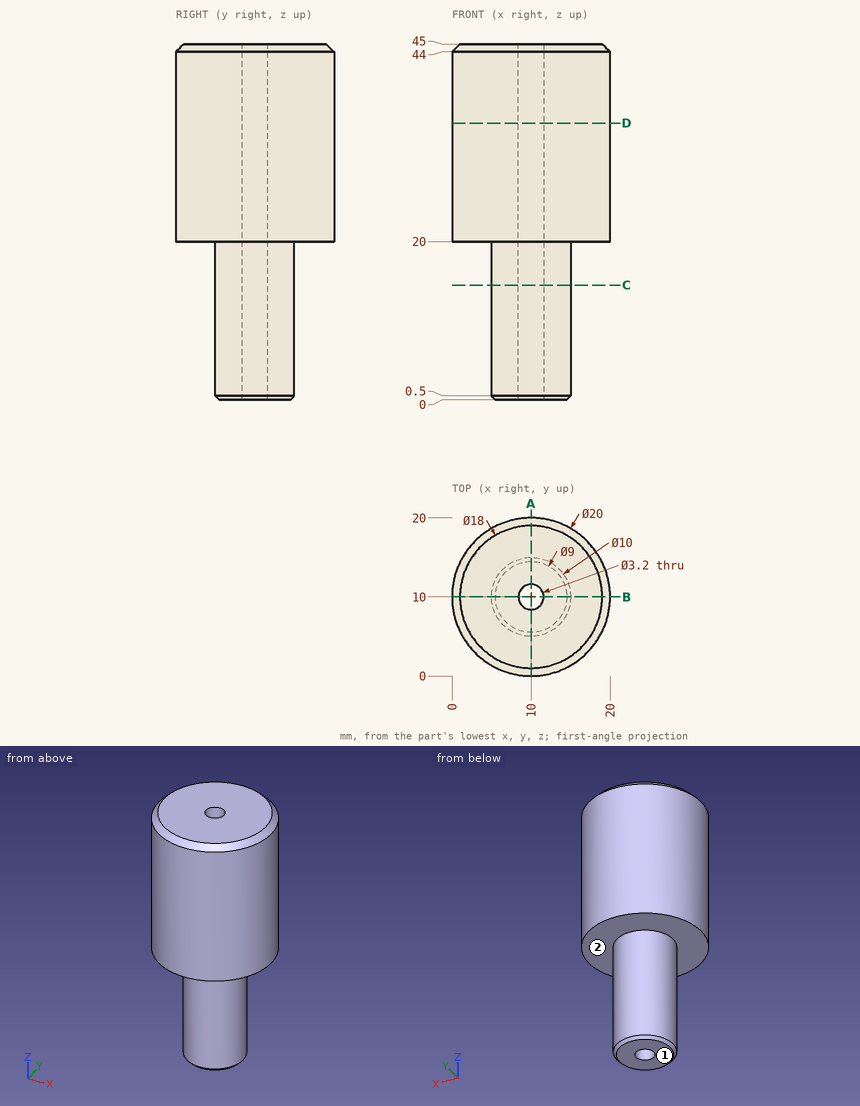
Study the drawing (mm; zero at the part's minimum x, y, z) and answer. A direction names the side the tool comes from. Give positions to 0.01 mm unless a question says otherwise; leave off trailing zeros. Order: outer loops, then holes, each group sorted by start corner. A loop starts at its lowest first (then second) coordinate and runs counter-clockwise, first axis right, second up.
1) For the marked faces 1 and 2, determine the directions among +Z, -Z, +X, -X, +Y, -Y from which every point of the face is accessible in a straight line to the end or side of a thin tool.
Reported:
face 1: -Z, +X, -X, +Y, -Y
face 2: -Z
2) Find section D-D on z = 35. Write down the section's boundary in (x, y), then the cut area to 3 significant figures.
Reported:
outline: circle Ø20 at (10, 10); hole circle Ø3.2 at (10, 10)
area: 306 mm2
3) Find section A-A on x = 10. Write down the section's boundary in (y, z), then the cut area to 3 significant figures.
Reported:
outline: (0, 20) - (5, 20) - (5, 0.5) - (5.5, 0) - (8.4, 0) - (8.4, 45) - (1, 45) - (0, 44) - close; (11.6, 0) - (14.5, 0) - (15, 0.5) - (15, 20) - (20, 20) - (20, 44) - (19, 45) - (11.6, 45) - close
area: 555 mm2
4) Consider line 1 along Y through (x, z) = (10, 22); line 2 along X through (y, z) = (9.25, 31); line 3 along Z through (x, y) = (3.5, 13). Determine where each line is inside the solid, lowest interval first.
Reported:
line 1: y = 0 to 8.4, 11.6 to 20
line 2: x = 0.03 to 8.59, 11.41 to 19.97
line 3: z = 20 to 45
5) Find section C-C on z = 14.5. Write down the section's boundary in (x, y), then the cut area to 3 significant figures.
Reported:
outline: circle Ø10 at (10, 10); hole circle Ø3.2 at (10, 10)
area: 70.5 mm2
6) Given P1, Ø8, axis at x = 16, z = 21.5, coming from the -Y side; P2, Ø5, axis at x = 16.5, z = 32.5, coming from the +Y side; P3, Ø1.5, axis at y = 10.5, z = 12, coming from the +X side, each flat-ended and moving along its own axis, determine where each tip first touches the part or whether it passes through.
Reported:
P1: stops at y = 0.2
P2: stops at y = 19.17
P3: stops at x = 15
